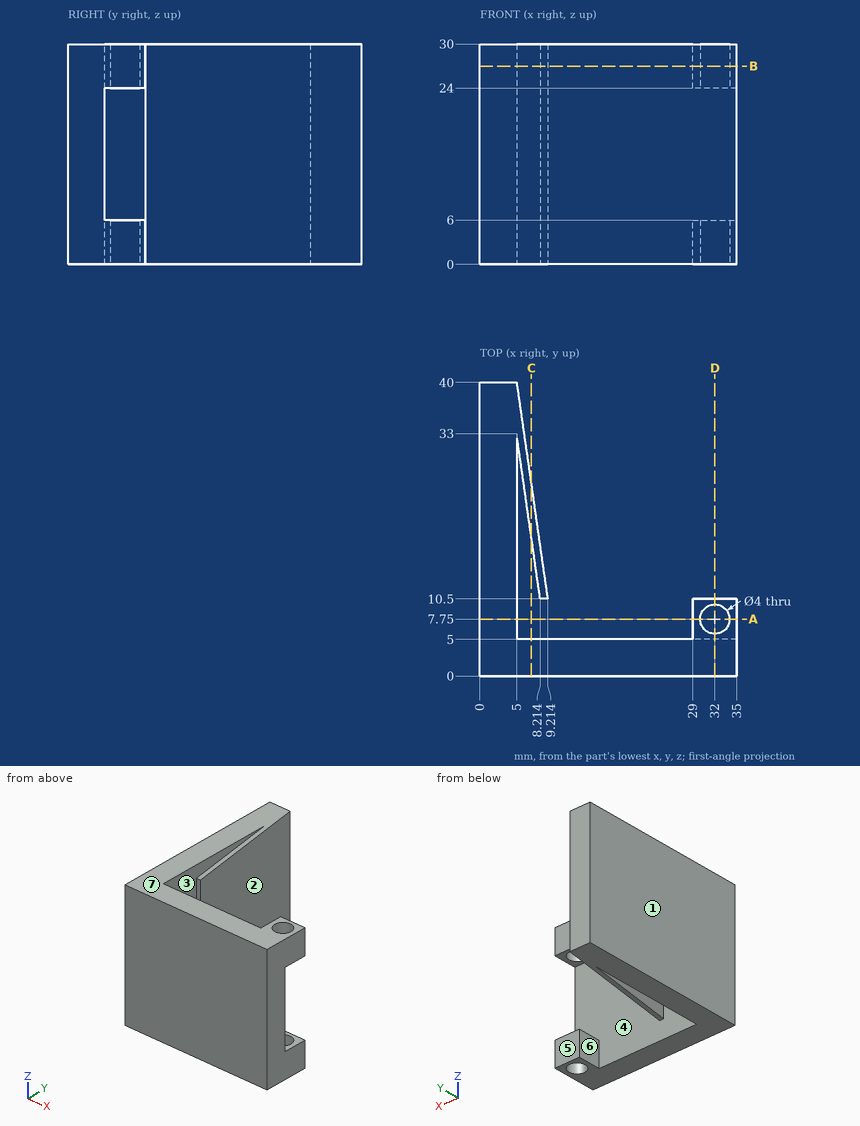
Print and shaded views of the part. All mm, measured from the part's lowest x, y and z. A direction names the side the tool comes from. Coordinates: 2 decimals unless noted, no trailing zeros. Write each loop counter-clockwise with the first axis right and the second up, starting at its lowest first coordinate (ties: lowest second). Pieces come first, ordered by that corner, then holes.
(1) Drill centre lines: probe 1 along X at (y, z) = (7.75, 26); probe 2 along Y at (x, z) = (32, 25.3); probe 3 along X at (y, z) = (10, 25.5). Where is each one in solid material? Low to high.
(2) Flat gauge pins, fed straight in: pin 1 (3 mm diameter, centred on x = 31.5, z = 27.5, fed in from +Y); pin 2 (8 mm diameter, centred on x = 19.5, z = 26, fed in from +Y). Where does each tip first touch, or does it go through?
(3) 3-axis set-ups, long thin cutter, end or side, ignore diameter. For the marked faces 5, 6 and 7: which of +Z, -Z, +X, -X, +Y, -Y reach the whole face in a straight line?
(4) Two-plate mould, pull along X, no slides. Class the marked faces 1, 2, 3 and 4: +X half, -X half, draft (parallel to the pull), parting line (faces both ways), or undercut.
(5) Cut at D-D, the plane x = 32. List the corners of the cut face in (y, z), and give its area (3 significant figures).
(6) Cut at A-A, the plane y = 7.75. List the corners of the cut face in (x, z).
(7) Cut at B-B, the plane z = 27. List the corners of the cut face in (x, y).
(8) Cut at C-C, the plane x = 7. List the corners of the cut face in (y, z), and give its area (3 significant figures).
Geometry says:
1. probe 1: x = 0 to 5, 29 to 30, 34 to 35
1. probe 2: y = 0 to 5.75, 9.75 to 10.5
1. probe 3: x = 0 to 5, 29 to 35
2. pin 1: stops at y = 10.5
2. pin 2: stops at y = 5
3. face 5: +Z, -Z, +X, +Y
3. face 6: +Z, -Z, +Y
3. face 7: +Z, +X, -X, +Y, -Y
4. face 1: -X half
4. face 2: +X half
4. face 3: undercut
4. face 4: undercut
5. outline: (0, 0) - (5.75, 0) - (5.75, 6) - (5, 6) - (5, 24) - (5.75, 24) - (5.75, 30) - (0, 30) - close; (9.75, 0) - (10.5, 0) - (10.5, 6) - (9.75, 6) - close; (9.75, 24) - (10.5, 24) - (10.5, 30) - (9.75, 30) - close
5. area: 168 mm2
6. outline: (0, 0) - (5, 0) - (5, 30) - (0, 30) - close; (29, 0) - (30, 0) - (30, 6) - (29, 6) - close; (29, 24) - (30, 24) - (30, 30) - (29, 30) - close; (34, 0) - (35, 0) - (35, 6) - (34, 6) - close; (34, 24) - (35, 24) - (35, 30) - (34, 30) - close
7. outline: (0, 0) - (35, 0) - (35, 10.5) - (29, 10.5) - (29, 5) - (5, 5) - (5, 33) - (8.21, 10.5) - (9.21, 10.5) - (5, 40) - (0, 40) - close; hole circle Ø4 at (32, 7.75)
8. outline: (0, 0) - (5, 0) - (5, 30) - (0, 30) - close; (19, 0) - (26, 0) - (26, 30) - (19, 30) - close
8. area: 360 mm2
